```python
from build123d import *

# Parameters (mm, degrees)
ESBO_O1_R                = 2.25
RESSALTO_EXTRUS_O1_DEPTH = 1
ESBO_O2_R                = 2.5
RESSALTO_EXTRUS_O2_DEPTH = 8
ESBO_O3_W                = 14
ESBO_O3_H                = 25.5
CORTE_EXTRUS_O1_DEPTH    = 56.463952257
ESBO_O5_R                = 12.5
ESBO_O5_R_2              = 2.5
RESSALTO_EXTRUS_O3_DEPTH = 6.5
FILETE1_R                = 3
ESBO_O6_R                = 2.5
ESBO_O6_R_2              = 2
RESSALTO_EXTRUS_O4_DEPTH = 8.5
FILETE2_R                = 2.5
FILETE3_R                = 15


# Some blends are built 0.0001 mm under size
with BuildPart() as part:
    # Esbo_o1 → Ressalto-extrus_o1 (new body)
    with BuildSketch(Plane(origin=(0, 0, 0), x_dir=(1, 0, 0), z_dir=(0, 1, 0))):
        with BuildLine():
            Line((2, 0), (30, 0))
            ThreePointArc((30, 0), (31.414213562, 0.585786438), (32, 2))
            Line((32, 2), (32, 35))
            ThreePointArc((32, 35), (31.414213562, 36.414213562), (30, 37))
            Line((30, 37), (2, 37))
            ThreePointArc((2, 37), (0.585786438, 36.414213562), (0, 35))
            Line((0, 35), (0, 2))
            ThreePointArc((0, 2), (0.585786438, 0.585786438), (2, 0))
        make_face()
        with Locations(Location((4, 33.5, 0), (0, 0, 270))):
            Circle(ESBO_O1_R, mode=Mode.SUBTRACT)
        with Locations(Location((28, 33.5, 0), (0, 0, 270))):
            Circle(ESBO_O1_R, mode=Mode.SUBTRACT)
        with Locations(Location((4, 3.5, 0), (0, 0, 270))):
            Circle(ESBO_O1_R, mode=Mode.SUBTRACT)
        with Locations(Location((28, 3.5, 0), (0, 0, 270))):
            Circle(ESBO_O1_R, mode=Mode.SUBTRACT)
    extrude(amount=RESSALTO_EXTRUS_O1_DEPTH)

    # Esbo_o2 → Ressalto-extrus_o2 (add, symmetric)
    with BuildSketch(Plane(origin=(16, 0, 0), x_dir=(0, 0, -1), z_dir=(1, 0, 0))):
        with BuildLine():
            Line((1, 22.5), (1, 4))
            Line((1, 4), (6, 4))
            Line((6, 4), (6, 1))
            Line((6, 1), (31, 1))
            Line((31, 1), (31, 4))
            Line((31, 4), (9.581688719, 25.988768539))
            ThreePointArc((9.581688719, 25.988768539), (4.116976314, 27.131870227), (1, 22.5))
        make_face()
        with Locations((6, 22.5)):
            Circle(ESBO_O2_R, mode=Mode.SUBTRACT)
    extrude(amount=RESSALTO_EXTRUS_O2_DEPTH, both=True)

    # Esbo_o3 → Corte-extrus_o1 (cut, through all)
    with BuildSketch(Plane.XY.offset(-1)):
        with Locations((16, 14.75)):
            Rectangle(ESBO_O3_W, ESBO_O3_H)
    extrude(amount=-CORTE_EXTRUS_O1_DEPTH, mode=Mode.SUBTRACT)



with BuildPart() as body_2:
    # Esbo_o5 → Ressalto-extrus_o3 (new, symmetric)
    with BuildSketch(Plane(origin=(16, 0, 0), x_dir=(0, 0, -1), z_dir=(1, 0, 0))):
        with Locations(Location((6, 22.5, 0), (0, 0, 180))):
            Circle(ESBO_O5_R)
        with Locations(Location((6, 22.5, 0), (0, 0, 270))):
            Circle(ESBO_O5_R_2, mode=Mode.SUBTRACT)
    extrude(amount=RESSALTO_EXTRUS_O3_DEPTH, both=True)

    # Filete1
    filete1_edges = [body_2.edges().sort_by_distance(p)[0] for p in [
        (9.5, 22.5, -18.5),
        (22.5, 22.5, -18.5),
    ]]
    fillet(filete1_edges, radius=FILETE1_R)


with BuildPart() as part_1:
    add(part.part)

    add(body_2.part)  # Ressalto-extrus_o4 merges body 2
    # Esbo_o6 → Ressalto-extrus_o4 (add, symmetric)
    with BuildSketch(Plane(origin=(16, 0, 0), x_dir=(0, 0, -1), z_dir=(1, 0, 0))):
        with Locations(Location((6, 22.5, 0), (0, 0, 270))):
            Circle(ESBO_O6_R)
        with Locations((6, 22.5)):
            Circle(ESBO_O6_R_2, mode=Mode.SUBTRACT)
    extrude(amount=RESSALTO_EXTRUS_O4_DEPTH, both=True)

    # Filete2
    filete2_edges = [part_1.edges().sort_by_distance(p)[0] for p in [
        (23.5, 4, -6),
        (8.5, 4, -1),
        (23.5, 4, -1),
    ]]
    fillet(filete2_edges, radius=FILETE2_R - 0.0001)  # a hair under: the kernel refuses the full size

    # Filete3
    # the kernel refuses this fillet: 15 mm, written as the material it takes off along each edge
    with BuildSketch(Plane(origin=(37.735072013, 4, -31), x_dir=(0, -1, 0), z_dir=(-1, 0, 0))) as filete3_piece_1:
        with BuildLine():
            CenterArc((6.530725419, 14.578545127), FILETE3_R, 225.752939657, 30.632936919)
            Line((-3.935580199, 3.83347897), (0, 0))
            Line((0, 0), (3, 0))
        make_face()
    extrude(amount=28.470144026, mode=Mode.SUBTRACT)
    with BuildSketch(Plane(origin=(22.735072013, 4, -31), x_dir=(0, 0.7163377438018307, 0.6977537078403117), z_dir=(-1, 0, 0))) as filete3_piece_2:
        with BuildLine():
            CenterArc((5.494028805, -15), FILETE3_R, 90, 30.632936919)
            Line((-2.149013231, -2.093261124), (0, 0))
            Line((0, 0), (5.494028805, 0))
        make_face()
    extrude(amount=28.470144026, mode=Mode.SUBTRACT)


solid = part_1.part
```
Input: part model. Units: mm. Frame: model coordinates. A direction names the side the tool comes from. Coordinates: 2 decimals unless noted, no trailing zeros. Write each loop counter-clockwise with the first axis right and the second up, starting at its lowest first coordinate (ties: lowest second). Pieces come first, ordered by that corner, then holes.
1) Material intervals for line 1 along X through (y, z) = (0.6, -33.5); line 2 along X through (y, z) = (7, -3.5); line 3 along Y through (x, z) = (6.5, -10.5), sorted ascending.
2) Pin query (flat end, axial travel): pin 1 Ø1.5 at (x, y) = (26.5, 23.5) entering from -Z; pin 2 Ø6.5 at (y, z) = (22.5, -6) entering from -X; pin 3 Ø4 at (x, y) = (12.5, 15.5) entering from +Z; pin 4 Ø21 at (y, z) = (14, -19.5) entering from +X. Return the tip coordinate at first contact, or that it passes through.
3) Mould query, pull axis Z, two halves, no side actions, for faces 1 (the cylindrical face through (23.51, 27.16, -4.19)), 2 (the flat face through (26, 1, -19)), 3 (the cylindrical face through (15.9, 21.3, -4.4)). Classes: pulls with the +Z half, pulls with the -Z half, needs draft (parallel to the pull), parting line crosses it, or undercut.
4) Set-up query: faces 4 (the flat face through (9.5, 24.5, -4)), 5 (the flat face through (16, 2, -18)), 6 (the cylindrical face through (24.3, 25, -6.1)), 7 (the flat face through (23.5, 14.6, -1)), 8 (the cylindrical face through (8.507, 4.713, -1.752)). Return all of +Z, -Z, +X, -X, +Y, -Y with unobstructed straight access to the full face (end or side cutting, diameter ignored); none if empty.
5) Section D-D on x = 15.5. Output: boundary loops of the cut face in (y, z).
6) Section A-A on x = 21. Output: boundary loops of the cut face in (y, z), and give its area (3 significant figures).
7) Section B-B on x = 28. Output: boundary loops of the cut face in (y, z), and give its area (3 significant figures).
8) Section C-C on z = -34. Output: boundary loops of the cut face in (x, y), and give its area (3 significant figures).
Check result:
1. line 1: x = 0 to 1.75, 6.25 to 25.75, 30.25 to 32
1. line 2: x = 8 to 9, 23 to 24
1. line 3: y = 0 to 1
2. pin 1: passes through
2. pin 2: stops at x = 7.5
2. pin 3: stops at z = 5.46
2. pin 4: stops at x = 24
3. face 1: parting line crosses it
3. face 2: needs draft
3. face 3: undercut
4. face 4: none
4. face 5: +Z, -Z
4. face 6: +X
4. face 7: +Z, +X, +Y
4. face 8: +Z, +X, -X
5. outline: (0, -37) - (1, -37) - (1, -31) arc R15 ccw to (2, -30.72) - (2, -5.95) arc R2.5 cw to (1.5, -6) - (1, -6) - (1, 0) - (0, 0) - close; circle Ø25 at (22.5, -6); hole circle Ø4 at (22.5, -6)
6. outline: (0, -37) - (1, -37) - (1, -31) arc R15 ccw to (2, -30.72) - (2, -5.95) arc R2.5 cw to (1.5, -6) - (1, -6) - (1, 0) - (0, 0) - close; circle Ø24.2 at (22.5, -6); hole circle Ø4 at (22.5, -6)
6. area: 509 mm2
7. outline: (0, -37) - (1, -37) - (1, -35.75) - (0, -35.75) - close; (0, -31.25) - (1, -31.25) - (1, -5.75) - (0, -5.75) - close; (0, -1.25) - (1, -1.25) - (1, 0) - (0, 0) - close
7. area: 28.0 mm2
8. outline: (0, 0) - (1.81, 0) - (1.81, 1) - (0, 1) - close; (6.19, 0) - (25.81, 0) - (25.81, 1) - (6.19, 1) - close; (30.19, 0) - (32, 0) - (32, 1) - (30.19, 1) - close
8. area: 23.2 mm2
